Read the model definition and answer for the solid it produces. Units are mm, in the model's axes. A direction names the side the tool comes from. Round coordinates to 2 decimals unless told otherwise and drop trailing zeros. Write each loop counter-clockwise with the first axis right and the second up, starting at its lowest first coordinate (ties: lowest second). Pieces come first, ordered by that corner, then holes. Notation, with made-up numbers: M 28.25,84 L 73.25,84 A24 ccw 73.25,104 Z; hole C -13.5,38 d9. An arc over 180 degrees is marked long. Use one line per item in the form item = value. Start each with the question number.
```python
from build123d import *

# Parameters (mm, degrees)
SKETCH1_W                       = 152.4
SKETCH1_H                       = 76.2
SKETCH1_R                       = 1.5875
BOSS_EXTRUDE1_DEPTH             = 19.05
SKETCH2_R                       = 4.7625
CUT_EXTRUDE1_DEPTH              = 6.35
F_1_4_0_25_DIAMETER_HOLE1_D     = 6.35
F_1_4_0_25_DIAMETER_HOLE1_DEPTH = 12.7
F_1_4_0_25_DIAMETER_HOLE1_TIP   = 1.907732465


with BuildPart() as part:
    # Sketch1 → Boss-Extrude1 (new body)
    with BuildSketch(Plane(origin=(0, 0, 0), x_dir=(0, 0, -1), z_dir=(1, 0, 0))):
        Rectangle(SKETCH1_W, SKETCH1_H)
        with Locations(Location((-38.1, 0, 0), (0, 0, 180))):
            Circle(SKETCH1_R, mode=Mode.SUBTRACT)
        with Locations(Location((-13.55, -7.860160654, 0), (0, 0, 180))):
            Circle(SKETCH1_R, mode=Mode.SUBTRACT)
        with Locations(Location((20.927, 1.096077429, 0), (0, 0, 180))):
            Circle(SKETCH1_R, mode=Mode.SUBTRACT)
        with Locations(Location((55.404, -9.873506971, 0), (0, 0, 180))):
            Circle(SKETCH1_R, mode=Mode.SUBTRACT)
    extrude(amount=BOSS_EXTRUDE1_DEPTH)

    # Sketch2 → Cut-Extrude1 (cut)
    with BuildSketch(Plane.ZY):
        with Locations((38.1, 0)):
            Circle(SKETCH2_R)
        with Locations((13.55, -7.860160654)):
            Circle(SKETCH2_R)
        with Locations((-20.927, 1.096077429)):
            Circle(SKETCH2_R)
        with Locations((-55.404, -9.873506971)):
            Circle(SKETCH2_R)
    extrude(amount=-CUT_EXTRUDE1_DEPTH, mode=Mode.SUBTRACT)

    # 1_4 _0.25_ Diameter Hole1
    with Locations(Plane.XZ.offset(38.1)):
        with Locations((9.525, -63.5), (9.525, 0), (9.525, 57.15)):
            Hole(F_1_4_0_25_DIAMETER_HOLE1_D / 2, depth=F_1_4_0_25_DIAMETER_HOLE1_DEPTH)
            with Locations((0, 0, -(F_1_4_0_25_DIAMETER_HOLE1_DEPTH + F_1_4_0_25_DIAMETER_HOLE1_TIP / 2))):  # 118° drill point
                Cone(0, F_1_4_0_25_DIAMETER_HOLE1_D / 2, F_1_4_0_25_DIAMETER_HOLE1_TIP, mode=Mode.SUBTRACT)


solid = part.part
```
Q1. For a pull along X with two mould halves and no side action, classify faces 1 (the face through (12.611, -9.265, -53.938)), 2 (the face through (9.82, -23.82, -63.04)), 3 (the face through (6.35, 0, 40)), 4 (the face through (19.05, 1, 1)) as +X half, -X half, draft (parallel to the pull), parting line (faces both ways), or undercut.
Q2. Find section A-A on z = 38.1. Write down the section's boundary in (x, y).
Q3. Straight lines are drawn through the part: line 1 (Z direction, x = 1.5, y = -10); line 2 (Y direction, x = 3, z = 38.1); line 3 (Y direction, x = 16.25, z = 13.55). For each, find the intervals that lie inside material, in ascending order. Write a range as [from, to].
Q4. Find section B-B on y = -29. Write down the section's boundary in (x, z) (3 decimals), and give its area (3 significant figures).
Q5. A tool of negligible diameter and unlimited length cuts with its end or side. For faces 5 (the face through (9.938, -31.661, -60.352)), 6 (the face through (6.35, -1, -21)), 7 (the face through (9, -1, 76.2)), from which of +Z, -Z, +X, -X, +Y, -Y can it reach the whole face along a straight path? Write none if from no direction.
Q6. Each of these flat-tipped pins is pushed along its axis until it touches: pin 1 Ø12.5 at (y, z) = (-7.86, 13.55) entering from -X; pin 2 Ø8.5 at (y, z) = (0, 38.1) entering from -X. Where does it stop, or does it pass through?
Response:
q1.face_1 = draft
q1.face_2 = undercut
q1.face_3 = -X half
q1.face_4 = +X half
q2.outline = M 0,-38.1 L 19.05,-38.1 L 19.05,-1.59 L 6.35,-1.59 L 6.35,-4.76 L 0,-4.76 Z; M 0,4.76 L 6.35,4.76 L 6.35,1.59 L 19.05,1.59 L 19.05,38.1 L 0,38.1 Z
q3.line_1 = [-76.2, -60.16], [-50.64, 9.3], [17.8, 76.2]
q3.line_2 = [-38.1, -4.76], [4.76, 38.1]
q3.line_3 = [-38.1, -9.45], [-6.27, 38.1]
q4.outline = M 0,-76.2 L 19.05,-76.2 L 19.05,76.2 L 0,76.2 Z; hole C 9.525,-63.5 d6.35; hole C 9.525,0 d6.35; hole C 9.525,57.15 d6.35
q4.area = 2,810 mm²
q5.face_5 = -Y
q5.face_6 = -X
q5.face_7 = +Z, +X, -X, +Y, -Y
q6.pin_1 = 0
q6.pin_2 = 6.35
